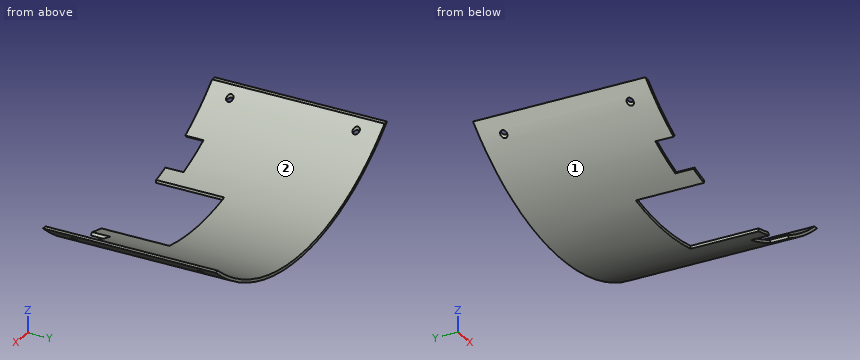
```python
from build123d import *

# Parameters (mm, degrees)
CURVED_PLATE_DEPTH      = 190
IR_CUTOUT_DEPTH         = 20
CHARGERBOX_CUTOUT_REACH = 67.75
SKETCH3_W               = 112
SKETCH3_H               = 75
SKETCH5_R               = 3.5687
MOUNTING_HOLES_DEPTH    = 66.75


with BuildPart() as part:
    # Sketch1 → Curved Plate (new body)
    with BuildSketch(Plane(origin=(0, 0, 0), x_dir=(1, 0, 0), z_dir=(0, 1, 0))):
        with BuildLine():
            Line((170.139573777, 0), (175, 0))
            ThreePointArc((175, 0), (0, 65.75), (-175, 0))
            Line((-175, 0), (-170.139573777, 0))
            ThreePointArc((-170.139573777, 0), (0, 62.575), (170.139573777, 0))
        make_face()
    extrude(amount=CURVED_PLATE_DEPTH)

    # Sketch2 → IR Cutout (cut)
    with BuildSketch(Plane(origin=(0, 0, 0), x_dir=(1, 0, 0), z_dir=(0, 1, 0))):
        with BuildLine():
            Line((-117.762328859, 38.234983169), (-105.521942389, 25.994596699))
            Line((-105.521942389, 25.994596699), (-101.986408483, 22.459062793))
            Line((-101.986408483, 22.459062793), (-73.702137236, 50.743334041))
            Line((-73.702137236, 50.743334041), (-77.237671141, 54.278867947))
            ThreePointArc((-77.237671141, 54.278867947), (-97.829451392, 47.089074697), (-117.762328859, 38.234983169))
        make_face()
        with BuildLine():
            Line((77.237671141, 54.278867947), (73.702137236, 50.743334041))
            Line((73.702137236, 50.743334041), (101.986408483, 22.459062793))
            Line((101.986408483, 22.459062793), (105.521942389, 25.994596699))
            Line((105.521942389, 25.994596699), (117.762328859, 38.234983169))
            ThreePointArc((117.762328859, 38.234983169), (97.829451392, 47.089074697), (77.237671141, 54.278867947))
        make_face()
    extrude(amount=IR_CUTOUT_DEPTH, mode=Mode.SUBTRACT)

    # Sketch3 → ChargerBox Cutout (cut, up to next)
    with BuildSketch(Plane.XY, mode=Mode.PRIVATE) as chargerbox_cutout_sk1:
        with Locations((0, 37.5)):
            Rectangle(SKETCH3_W, SKETCH3_H)
    chargerbox_cutout_tool1 = extrude(chargerbox_cutout_sk1.sketch, amount=-CHARGERBOX_CUTOUT_REACH, mode=Mode.PRIVATE) & part.part
    add(chargerbox_cutout_tool1.solids().sort_by_distance((0, 37.5, 0))[0], mode=Mode.SUBTRACT)

    # Sketch5 → Mounting Holes (cut, through all)
    with BuildSketch(Plane.XY):
        with Locations((-159.125, 164.6)):
            Circle(SKETCH5_R)
        with Locations((-159.125, 25.4)):
            Circle(SKETCH5_R)
        with Locations((159.125, 25.4)):
            Circle(SKETCH5_R)
        with Locations((159.125, 164.6)):
            Circle(SKETCH5_R)
    extrude(amount=-MOUNTING_HOLES_DEPTH, mode=Mode.SUBTRACT)


solid = part.part
```
Here's how the part is built. I have some questions about the finished solid (model axes, mm). Face numbers are marked on the shaded views. Round coordinates to 2 decimals unless told otherwise and drop trailing zeros. Loops run counter-clockwise (first coordinate to the right, second up) from the corner with the lowest first, then second, coordinate; pieces in that order, holes last.
1. Suppose I cut it at A-A, the plane z = -32.5. Please give me the cut outline in (x, y).
Answers:
outline: (-128.72, 0) - (-122.03, 0) - (-122.03, 190) - (-128.72, 190) - close; (122.03, 0) - (128.72, 0) - (128.72, 190) - (122.03, 190) - close
2. Suppose I cut it at C-C, the plane y = 164.6. Please give me the cut outline in (x, z).
Answers:
outline: (-175, 0) arc R265.76 ccw to (-162.69, -10.13) - (-162.69, -6.1) arc R262.59 cw to (-170.14, 0) - close; (-155.56, -15.47) arc R265.76 ccw to (155.56, -15.47) - (155.56, -11.54) arc R262.59 cw to (-155.56, -11.54) - close; (162.69, -10.13) arc R265.76 ccw to (175, 0) - (170.14, 0) arc R262.59 cw to (162.69, -6.1) - close
3. Thinking about a two-plate mould opening in X: for the marked faces 1 and 2, which applies, released by +X, released by -X, zero draft, split by the parting line, or undercut?
Answers:
face 1: split by the parting line
face 2: undercut
4. If I drill on probe 1 along Y at (x, z) = (-158, -10.5); probe 2 along X at (y, z) = (181, -16.5); probe 3 along X at (y, z) = (16, -11.5), over which ranges is the centre line in solid material (lowest first)?
Answers:
probe 1: y = 0 to 22.01, 28.79 to 161.21, 167.99 to 190
probe 2: x = -154.12 to -148.58, 148.58 to 154.12
probe 3: x = -160.91 to -155.61, 155.61 to 160.91
5. Suppose I cut it at B-B, the plane y = 25.4. Please give me the cut outline in (x, z).
Answers:
outline: (-175, 0) arc R265.76 ccw to (-162.69, -10.13) - (-162.69, -6.1) arc R262.59 cw to (-170.14, 0) - close; (-155.56, -15.47) arc R265.76 ccw to (-56, -59.78) - (-56, -56.53) arc R262.59 cw to (-155.56, -11.54) - close; (56, -59.78) arc R265.76 ccw to (155.56, -15.47) - (155.56, -11.54) arc R262.59 cw to (56, -56.53) - close; (162.69, -10.13) arc R265.76 ccw to (175, 0) - (170.14, 0) arc R262.59 cw to (162.69, -6.1) - close
6. Suppose I cut it at D-D, the plane x = -142. Please give me the cut outline in (y, z), and give its area (3 significant figures).
Answers:
outline: (0, -24.63) - (190, -24.63) - (190, -20.87) - (0, -20.87) - close
area: 715 mm2
7. Will these pins go through, and if not, where does the flat tip stop? pin 1 (6 mm diameter, centred on x = 84.5, y = 45.5, fed in from +Z); pin 2 (7.5 mm diameter, centred on x = 3, z = -61, fed in from -Y); pin 3 (9 mm diameter, centred on x = 86, z = -48, fed in from -Y); pin 4 (4.5 mm diameter, centred on x = 159.125, y = 164.6, fed in from -Z).
Answers:
pin 1: stops at z = -47.57
pin 2: stops at y = 75
pin 3: stops at y = 20
pin 4: passes through
